Autodesk Inventor part; units mm, degrees
ref_plane "Work Plane1" through (6.0312, 0, 0) normal (0, 0, -1) x (-1, 0, 0)
ref_plane "YZ Plane" through (0, 0, 0) normal (1, 0, 0) x (0, 1, 0)
ref_plane "XZ Plane" through (0, 0, 0) normal (0, 1, 0) x (-1, 0, 0)
sketch "Skizze1" plane through (0, 0, 0) normal (0, 0, 1) x (1, 0, 0)
  line L0 (0, 0) -> (-4, 0)
  line L1 (0, 0) -> (0, 8)
  line L2 (0, 8) -> (-3.5, 8)
  line L3 (-3.5, 8) -> (-3.5, 4.5)
  line L4 (-4, 4) -> (-4, 4)
  line L5 (-4, 4) -> (-4, 0)
  arc A0 (-4, 4) -> (-3.5, 4.5) centre (-4, 4.5) ccw
  dimension "d0" = 0.5
  dimension "d1" = 4
  dimension "d2" = 16
  dimension "d3" = 8
revolve "Körper" add sketch "Skizze1" angle 360 about axis through (0, 0, 0) along (-1, 0, 0)
sketch "Skizze2" plane through (-4, 0, 0) normal (-1, 0, 0) x (0, 0, 1)
  circle A0 centre (0, 0) radius 8
  line L0 (0, 0) -> (0, 8) construction
  line L1 (-0.25, 7.9961) -> (0, 7.7461)
  line L2 (0.25, 7.9961) -> (0, 7.7461)
  arc A1 (0.25, 7.9961) -> (-0.25, 7.9961) centre (0, 0) ccw
  circle A2 centre (0, 0) radius 4
  dimension "d4" = 90
  dimension "d5" = 0.25
chamfer "Fase1" distance 0.4 angle 45 1 edges at (0, -8, 0) measured on face at (0, 3.2134, 0.792)
chamfer "Fase2" distance 0.4 angle 45 1 edges at (-3.5, -8, 0) measured on face at (-3.5, 6.7558, 0.6382)
extrude "Nut1" [suppressed]
pattern_circular "Nuten1" [suppressed]
hole "Gewinde" at (-4, 0, 0) direction (1, 0, 0) diameter 3.242 end through all
chamfer "Fase3" distance 0.3789 angle 30 1 edges at (-4, 0, -1.621) measured on face at (-4, 3.1643, 0.3842)
ref_plane "Work Plane1" through (6.0312, 0, 0) normal (0, 0, -1) x (-1, 0, 0)
equation "\"d5\" = 0.5 * T"
equation "\"d13\" = PHH"
equation "\"d15\" = FAWI"
equation "\"d36\" = PHH"
equation "\"d23\" = PHH"
equation "\"d24\" = FAWI"
equation "\"d37\" = PHH"
equation "\"d10\" = -0.5 * GD1 + 0.5 * NND"
equation "\"d38\" = -0.5 * GD1 + 0.5 * NND"
equation "\"d0\" = RR"
equation "\"d1\" = KOH"
equation "\"d2\" = KOD"
equation "\"d3\" = BDM"
equation "\"FAWI\" = 45deg"
equation "\"T\" = 0.5"
equation "\"NND\" = 4"
equation "\"KOD\" = 16"
equation "\"KOH\" = 4"
equation "\"KOH1\" = 3.5"
equation "\"BDM\" = 8"
equation "\"PHH\" = 0.4"
equation "\"RR\" = 0.5"
equation "\"GUL\" = 0.541266 * PTC"
equation "\"THREADDIA\" = 4"
equation "\"TOA\" = 30deg"
equation "\"PTC\" = 0.7"
equation "\"GAL\" = 0.541266 * PTC"
properties part number "DIN 467 - M4" material "Stahl, weich"
Design review of the part built by this model. Coordinates are the model's own, in mm. Give positions to 0.01 mm unless a question says otherwise; leave off trailing zeros. Write each loop counter-clockwise with the first axis right and the second up, starting at its lowest first coordinate (ties: lowest second). Pieces come first, ordered by that corner, then holes.
(1) Mouldability with a two-part tool opening along Y and no side actions: class faces 1 (the face through (-1.864, 1.438, 0.748)), 2 (the face through (-3.5, 3.3, 3.3)), 3 (the face through (-1.77, -1.73, 7.81)) as +Y half, -Y half, draft (parallel to the pull), parting line (faces both ways), or undercut.
Checked values:
face 1: undercut
face 2: draft
face 3: parting line
(2) Add section D-D (x = -3.3). Give the boundary of the cut face in (y, z).
Checked values:
outline: circle Ø15.6 at (0, 0); hole circle Ø3.24 at (0, 0)
(3) Clearance check with flat-ended pins moving along their axes: pin 1 Ø1.5 at (x, z) = (-3, -3) entering from +Y; pin 2 Ø1.9 at (y, z) = (0, 0) entering from +X. State where each tip first meets the part, or that it passes through.
Checked values:
pin 1: stops at y = 7.68
pin 2: passes through
(4) Wall thickness on line 1 along Y through (x, z) = (-0.75, 0); line 2 along X through (y, z) = (-2.5, -7): over which ranges is each line inside the solid? List them lowest first.
Checked values:
line 1: y = -8 to -1.62, 1.62 to 8
line 2: x = -3.5 to 0
(5) Add section A-A (z = 0). Give the boundary of the cut face in (x, y).
Checked values:
outline: (-4, -4) arc R0.5 cw to (-3.5, -4.5) - (-3.5, -7.6) - (-3.1, -8) - (-0.4, -8) - (0, -7.6) - (0, -1.62) - (-3.78, -1.62) - (-4, -2) - close; (-4, 2) - (-3.78, 1.62) - (0, 1.62) - (0, 7.6) - (-0.4, 8) - (-3.1, 8) - (-3.5, 7.6) - (-3.5, 4.5) arc R0.5 cw to (-4, 4) - close
(6) Add section C-C (x = -2.1). Give the boundary of the cut face in (y, z).
Checked values:
outline: circle Ø16 at (0, 0); hole circle Ø3.24 at (0, 0)
